For this review, use the dimensioned drawing (mm, ordinates from the lowest corner) and the shaded views. Round coordinates to 2 decimals unless told otherwise and drop trailing zeros. Write each loop counter-clockwise with the first axis right and the second up, starting at its lowest first coordinate (ties: lowest second). Pieces come first, ordered by that corner, then holes. Notation, with made-up numbers: M 70.5,41.5 L 123.5,41.5 A21 ccw 123.5,78.5 Z; hole C -34,-31 d7. An arc over 180 degrees is marked long. Write each question's results on one line, items separated by ' | '. Start each with the question number.
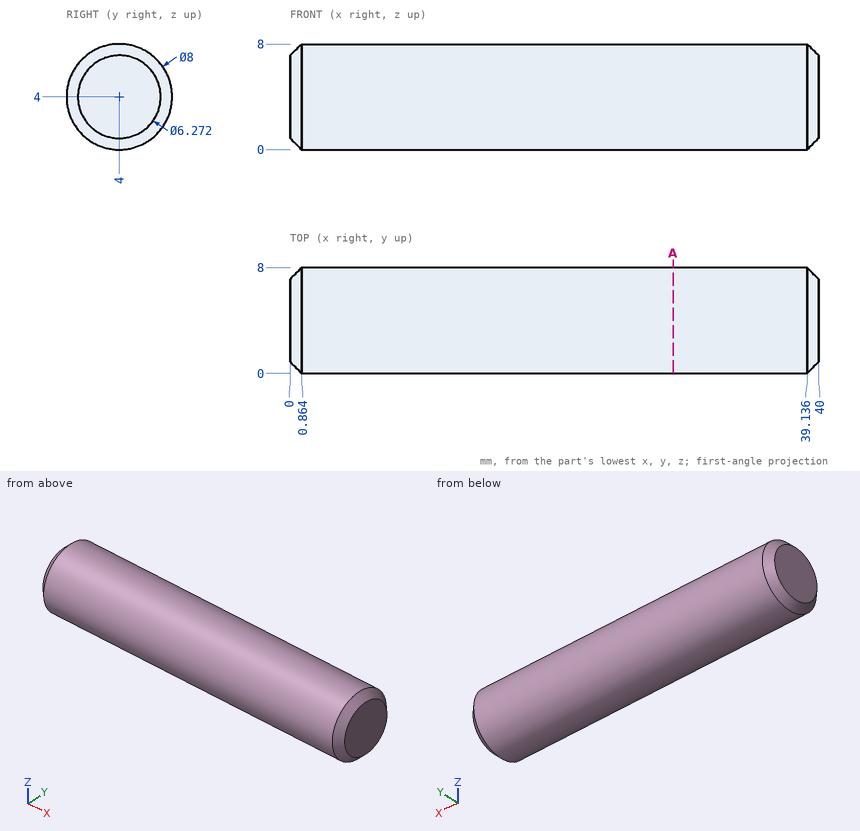
Item 1: For probe 1 along Z at (x, y) = (28, 3); probe 2 along Z at (x, y) = (32.5, 1.5); probe 3 along Y at (x, z) = (15, 1.75), list the stretches that pass through material, from the lowest coordinate up.
Item 2: Insertion check: P1, Ø4, axis at x = 29, z = 2.5, coming from the -Y side; P2, Ø4, axis at x = 26, z = 7, coming from the +Y side; P3, Ø1.5, axis at x = 35, z = 6.5, coming from the +Y side. Each pin has a flat end and moves straight along its axis. Give the tip position at first contact, or say it passes through.
Item 3: We need section A-A on x = 29. State the section outline as (y, z) points.
Numbers:
1) probe 1: z = 0.13 to 7.87 | probe 2: z = 0.88 to 7.12 | probe 3: y = 0.69 to 7.31
2) P1: stops at y = 0 | P2: stops at y = 7.87 | P3: stops at y = 7.6
3) outline: C 4,4 d8
